Verification items for the finished model (mm, model axes). A direction names the side the tool comes from. Coordinates: 2 decimals unless noted, no trailing zeros. Loops run counter-clockwise (first coordinate to the right, second up) from the corner with the lowest first, then second, coordinate; pieces in that order, holes last. Notation, with made-up numbers: (27, 78.5) - (79, 78.5) arc R10 ccw to (79, 95.5) - close; hole circle Ø5 at (83.25, 15.25). An arc over 180 degrees is marked (long way). Answer as CSV lines item,"result". Start each with the question number.
1. Gauge pin test, flat ends, axial feed: P1, Ø4, axis at y = -97.5, z = 42.5, coming from the -X side; P2, Ø15, axis at y = 85.5, z = 16.5, coming from the -X side; P3, Ø1.5, axis at y = 47, z = 37, coming from the +X side; P4, Ø4, axis at x = 35, y = 13, coming from the -Z side. Record the tip position at first contact, or that the pin passes through.
2. Cross-section at C-C (y = -39.5). Enter the section's corners in (x, z).
3. Set-up check for faces 1 (the flat face through (85.57, -30.43, 25.35)), 2 (the cylindrical face through (9.18, -28.56, 24.65)), 3 (the cylindrical face through (-9.18, 28.56, 24.65)): record each of +Z, -Z, +X, -X, +Y, -Y from which the full face is reachable in a straight line by a thin tool's end or side.
4. Cross-section at A-A (y = 0). Enter the section's corners in (x, z), plus the area to 3 significant figures.
5. Cross-section at B-B (x = 101.5). Enter the section's corners in (y, z), plus the area to 3 significant figures.
6. Cross-section at D-D (y = 78.5). Enter the section's corners in (x, z).
7. Material ranges on line 1 (Y direction, x = 0, z = 24); line 2 (Y direction, x = -86, z = 18.5); line 3 (X direction, y = 0, z = 31), recorded low to high. Write a range as [from, to].
8. Release check for a two-part mould opening along X. For faces 4 (the flat face through (-87.12, 25.68, 25.35)), 5 (the flat face through (55.4, 72, 25.3)) record: pulls with the +X half, pulls with the -X half, needs draft (parallel to the pull), parting line crosses it, or undercut.
```python
from build123d import *

# Parameters (mm, degrees)
SKETCH_1_R               = 30
EXTRUDE_1_DEPTH          = 50
CUT_EXTRUDE_1_DEPTH      = 66.574385243
EXTRUDE_2_REACH          = 191.209
EXTRUDE_2_END_RADIUS     = 30
SKETCH_3_W               = 5
SKETCH_3_H               = 50
PATTERN_CIRCULAR_1_COUNT = 10


with BuildPart() as part:
    # 草图1 → 凸台-拉伸1 (new body)
    with BuildSketch(Plane.XY):
        Circle(SKETCH_1_R)
    extrude(amount=EXTRUDE_1_DEPTH)

    # 草图2 → 切除-拉伸1 (cut, through all)
    with BuildSketch(Plane.XY.offset(50)):
        with BuildLine():
            Line((-3, 18), (3, 18))
            Line((3, 18), (3, 14.696938457))
            ThreePointArc((3, 14.696938457), (0, -15), (-3, 14.696938457))
            Line((-3, 14.696938457), (-3, 18))
        make_face()
    extrude(amount=-CUT_EXTRUDE_1_DEPTH, mode=Mode.SUBTRACT)

    # 凸台-拉伸2: up to this cylinder (the profile starts outside it)
    extrude_2_end = Plane(origin=(0, 0, 25), z_dir=(0, 0, -1)) * Cylinder(EXTRUDE_2_END_RADIUS, 443.418, mode=Mode.PRIVATE)
    # 草图3 → 凸台-拉伸2 (add, up to the surface)
    with BuildSketch(Plane(origin=(0, 150, 0), x_dir=(1, 0, 0), z_dir=(0, 1, 0)), mode=Mode.PRIVATE) as extrude_2_sk1:
        with Locations((0, -25)):
            Rectangle(SKETCH_3_W, SKETCH_3_H)
    extrude_2_tool1 = extrude(extrude_2_sk1.sketch, amount=-EXTRUDE_2_REACH, mode=Mode.PRIVATE) - extrude_2_end
    extrude_2 = extrude_2_tool1.solids().sort_by_distance((0, 150, 25))[0]
    add(extrude_2)

    # 阵列(圆周)1: 凸台-拉伸2 ×10 about axis
    pattern_circular_1_axis = Axis((0, 0, 0), (0, 0, 1))
    for i in range(1, PATTERN_CIRCULAR_1_COUNT):
        add(extrude_2.rotate(pattern_circular_1_axis, i * 360 / PATTERN_CIRCULAR_1_COUNT))


solid = part.part
```
Values follow:
1,P1,"stops at x = -75.38"
1,P2,"stops at x = -70.66"
1,P3,"stops at x = 142.69"
1,P4,"stops at z = 0"
2,outline,"(-129.66, 0) - (-113.48, 0) - (-113.48, 50) - (-129.66, 50) - close; (-31.79, 0) - (-25.61, 0) - (-25.61, 50) - (-31.79, 50) - close; (-2.5, 0) - (2.5, 0) - (2.5, 50) - (-2.5, 50) - close; (25.61, 0) - (31.79, 0) - (31.79, 50) - (25.61, 50) - close; (113.48, 0) - (129.66, 0) - (129.66, 50) - (113.48, 50) - close"
3,face 1,"+Z, -Z"
3,face 2,"+Z, -Z, -Y"
3,face 3,"+Z, -Z, +Y"
4,outline,"(-30, 0) - (-15, 0) - (-15, 50) - (-30, 50) - close; (15, 0) - (30, 0) - (30, 50) - (15, 50) - close"
4,area,"1,500 mm²"
5,outline,"(-35.61, 0) - (-30.35, 0) - (-30.35, 50) - (-35.61, 50) - close; (30.35, 0) - (35.61, 0) - (35.61, 50) - (30.35, 50) - close"
5,area,"526 mm²"
6,outline,"(-60.12, 0) - (-53.94, 0) - (-53.94, 50) - (-60.12, 50) - close; (-2.5, 0) - (2.5, 0) - (2.5, 50) - (-2.5, 50) - close; (53.94, 0) - (60.12, 0) - (60.12, 50) - (53.94, 50) - close"
7,line 1,"y = [-150, -15], [18, 150]"
7,line 2,"y = [-122.62, -114.12], [-30.57, -25.31], [25.31, 30.57], [114.12, 122.62]"
7,line 3,"x = [-30, -15], [15, 30]"
8,face 4,"pulls with the -X half"
8,face 5,"undercut"
